Read the model definition and answer for the solid it produces. Units are mm, in the model's axes. A direction names the side the tool comes from. Round coordinates to 2 decimals unless told otherwise and drop trailing zeros. Loops run counter-clockwise (first coordinate to the right, second up) from the corner with the lowest first, then second, coordinate; pieces in that order, holes last. Notation, with made-up numbers: (-29, -24.75) -> (-5, -24.75) arc R7 ccw to (-5, -11.75) -> close; hole circle Ø4 at (-20.75, 30.5). An arc over 180 degrees is marked (long way). Put each result on its own line as item: value.
Solid Edge part; units mm, degrees
sketch "Sketch1" plane through (0, 0, 0) normal (0, 0, 1) x (1, 0, 0)
  line L0 (4, 0) -> (4, 20)
  line L1 (0, 20) -> (4, 20)
  line L2 (0, 0) -> (0, 20)
  line L3 (0, 0) -> (0, -4.4)
  line L4 (0, -4.4) -> (7, -4.4)
  line L5 (7, -4.4) -> (7, 0)
  line L6 (7, 0) -> (4, 0)
revolve "RevolvedProtrusion1" add sketch "Sketch1" angle 360 about axis through (0, 0, 0) along (0, 1, 0)
sketch "Sketch2" plane through (0, 0, 0) normal (1, 0, 0) x (0, 1, 0)
  line L0 (-4.4, 3.3615) -> (-1.8, 3.3615)
  line L1 (0.1408, 0) -> (-1.8, 3.3615)
  line L2 (-4.4, 0) -> (0.1408, 0)
  line L3 (-4.4, 0) -> (-4.4, 3.3615)
revolve "RevolvedCutout1" cut sketch "Sketch2" angle 360 about axis through (0, -4.5, 0) along (0, 1, 0)
sketch "Sketch3" plane through (0, -4.4, 0) normal (0, -1, 0) x (0, 0, 1)
  circle A0 centre (0, 0) radius 3.3615
  line L0 (-2.5, -1.4434) -> (0, -2.8868)
  line L1 (0, -2.8868) -> (2.5, -1.4434)
  line L2 (2.5, -1.4434) -> (2.5, 1.4434)
  line L3 (2.5, 1.4434) -> (0, 2.8868)
  line L4 (0, 2.8868) -> (-2.5, 1.4434)
  line L5 (-2.5, 1.4434) -> (-2.5, -1.4434)
extrude "Protrusion1" add sketch "Sketch3" against normal up to next
sketch "Sketch4" plane through (0, 0, 0) normal (0, 0, 1) x (1, 0, 0)
  line L0 (-2.8868, -4.4) -> (0, -4.4)
  line L1 (0, -4.4) -> (0, -3.6265)
  line L2 (0, -3.6265) -> (-2.8868, -4.4)
revolve "RevolvedCutout2" cut sketch "Sketch4" angle 360 about axis through (0, -4.5, 0) along (0, 1, 0)
fillet "Round1" radius 0.4 1 edges at (0, 0, -4)
chamfer "倒斜角_2" distance 0.5333 angle 45 1 edges at (0, 20, -4)
cosmetic_thread "螺纹_3" thread depth 17.5
sketch "Sketch5" plane through (0, 0, 0) normal (0, 0, 1) x (1, 0, 0)
  arc A0 (-3.8153, -4.4) -> (-7, 0) centre (-2.3681, 0) cw
revolve "RevolvedCutout3" cut sketch "Sketch5" angle 360 about axis through (0, 0, 0) along (0, -1, 0) material side at (-6.1609, -2.7452, 0)
Item 1: The part is cut by section A-A (y = 6.5). Determine the outline of the cut face in (x, z).
Derived:
outline: circle Ø8 at (0, 0)
Item 2: Find the intervals of material crossed by line 1 along Z through (x, y) = (0, 11.5); line 2 along X through (y, z) = (13.75, 1.25), in increasing order.
Derived:
line 1: z = -4 to 4
line 2: x = -3.8 to 3.8
Item 3: Which of the six approach directions +Z, -Z, +X, -X, +Y, -Y give full straight-line access (tool end or side, diameter ignored) to faces 5 (the flat face through (0, 0, 5)), 6 (the flat face through (-3, -4.4, 1)), 7 (the flat face through (-2.155, -2.873, 1.268))?
Derived:
face 5: +Y
face 6: +Z, -Z, +X, -X, -Y
face 7: -Y
Item 4: Flat-ended cylindrical pins translate along their axes: pin 1 Ø3 at (x, y) = (0, -2.5) entering from -Z; pin 2 Ø3 at (y, z) = (16, -2.5) entering from -X; pin 3 Ø2 at (y, z) = (5.5, 3) entering from -X. Find the tip coordinate at first contact, or state that the pin passes through.
Derived:
pin 1: stops at z = -6.89
pin 2: stops at x = -3.87
pin 3: stops at x = -3.46
Item 5: For a pull along Z with two mould halves and no side action, classify faces 1 (the flat face through (0, -3, -2.5)), 2 (the flat face through (0, 20, 0)), 3 (the cylindrical face through (-0.867, 10.067, 3.905)), 4 (the conical face through (0.058, -4.337, 2.652)) as pulls with the +Z half, pulls with the -Z half, needs draft (parallel to the pull), parting line crosses it, or undercut.
Derived:
face 1: undercut
face 2: needs draft
face 3: parting line crosses it
face 4: undercut
